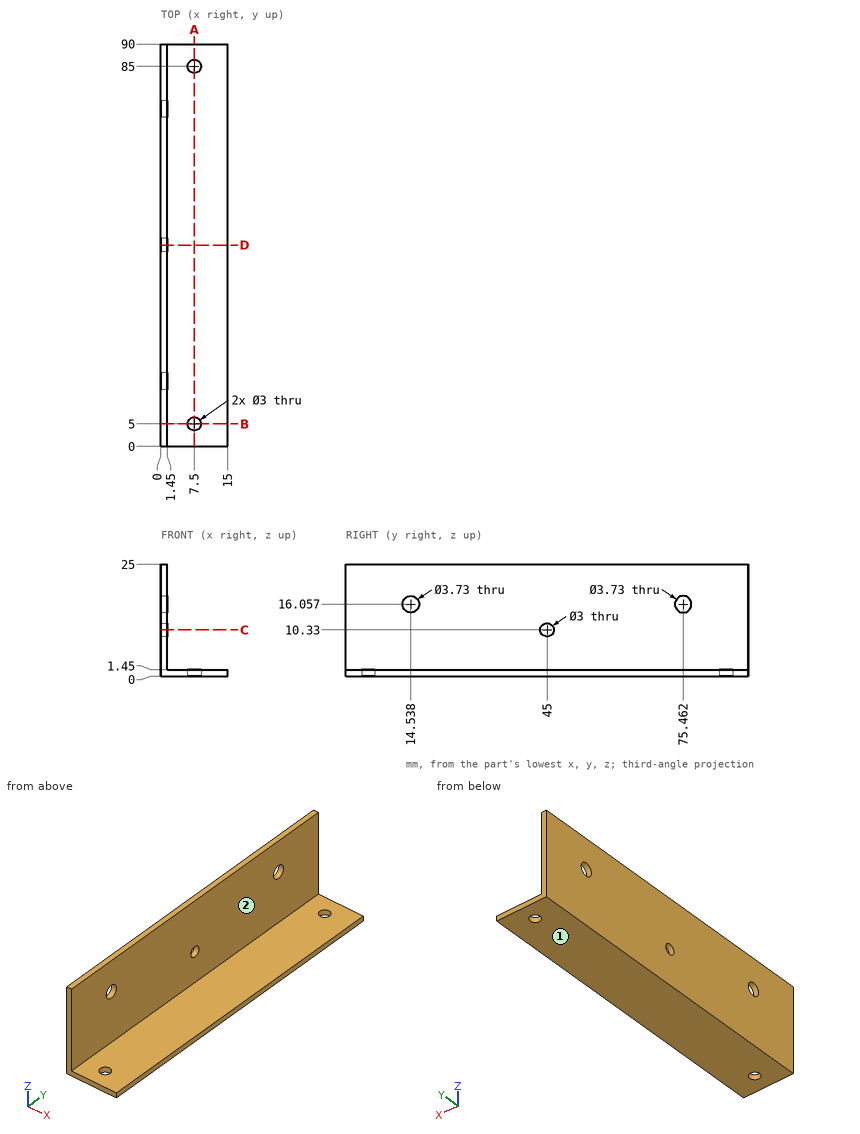
For this review, use the dimensioned drawing (mm, ordinates from the lowest corner) and the shaded views. A direction names the side the tool comes from. Give positions to 0.01 mm unless a question says otherwise; leave off trailing zeros. Order: outer loops, then holes, each group sorted by start corner. A loop starts at its lowest first (then second) coordinate and runs counter-clockwise, first axis right, second up. Notation, with made-up numbers: (-34, 71.25) - (2, 71.25) arc R35 cw to (2, 108.25) - close; hole circle Ø3 at (80.25, 12.5). An arc over 180 degrees is marked (long way). Write item = value, one per line. Start each with the question number.
Q1. We need section B-B on y = 5. State the section outline as (x, z) points.
Q2. We need section A-A on x = 7.5. State the section outline as (y, z) points.
Q3. Tool access review of the marked faces 1 and 2: name each direction out of +Z, -Z, +X, -X, +Y, -Y from which nothing blocks a thin tool from reaching the whole face with its end or side.
Q4. Clearance check with flat-ended pins moving along their axes: pin 1 Ø7 at (x, y) = (11, 62.5) entering from +Z; pin 2 Ø5 at (x, y) = (7.5, 85) entering from -Z; pin 3 Ø1.8 at (y, z) = (45, 10.33) entering from +X; pin 4 Ø12 at (y, z) = (69, 10) entering from +X. State where each tip first meets the part, or that it passes through.
Q5. To check wall thickness, follow L1, parallel to Y at x = 7.5, z = 0.65; L2, parallel to X at y = 85, z = 0.6; L3, parallel to Y at x = 1, z = 10.33. State the ranges of each line that lie inside material, in increasing order. Write a range as from..to.
Q6. We need section D-D on y = 45. State the section outline as (x, z) points, plus the area to 3 significant figures.
Q7. We need section C-C on z = 10.33. State the section outline as (x, y) points.
Working result:
q1.outline = (0, 0) - (6, 0) - (6, 1.45) - (1.45, 1.45) - (1.45, 25) - (0, 25) - close; (9, 0) - (15, 0) - (15, 1.45) - (9, 1.45) - close
q2.outline = (0, 0) - (3.5, 0) - (3.5, 1.45) - (0, 1.45) - close; (6.5, 0) - (83.5, 0) - (83.5, 1.45) - (6.5, 1.45) - close; (86.5, 0) - (90, 0) - (90, 1.45) - (86.5, 1.45) - close
q3.face_1 = -Z, +X, -X, +Y, -Y
q3.face_2 = +Z, +X, +Y, -Y
q4.pin_1 = 1.45
q4.pin_2 = 0
q4.pin_3 = through
q4.pin_4 = 1.45
q5.L1 = 0..3.5, 6.5..83.5, 86.5..90
q5.L2 = 0..6, 9..15
q5.L3 = 0..43.5, 46.5..90
q6.outline = (0, 0) - (15, 0) - (15, 1.45) - (1.45, 1.45) - (1.45, 8.83) - (0, 8.83) - close; (0, 11.83) - (1.45, 11.83) - (1.45, 25) - (0, 25) - close
q6.area = 51.5 mm²
q7.outline = (0, 0) - (1.45, 0) - (1.45, 43.5) - (0, 43.5) - close; (0, 46.5) - (1.45, 46.5) - (1.45, 90) - (0, 90) - close
